```python
from build123d import *

# Parameters (mm, degrees)
BOSS_EXTRUDE1_DEPTH = 52.34
SKETCH2_R           = 2.2
CUT_EXTRUDE1_DEPTH  = 80
SKETCH3_R           = 49.6
CUT_EXTRUDE2_DEPTH  = 30


with BuildPart() as part:
    # Sketch1 → Boss-Extrude1 (new body)
    with BuildSketch(Plane(origin=(0, 0, 0), x_dir=(1, 0, 0), z_dir=(0, 1, 0))):
        with BuildLine():
            ThreePointArc((-53.971636069, -1.75), (-38.183766184, -38.183766184), (-1.75, -53.971636069))
            Line((-1.75, -53.971636069), (-1.75, -52.271636069))
            Line((-1.75, -52.271636069), (1.75, -52.271636069))
            Line((1.75, -52.271636069), (1.75, -53.971636069))
            ThreePointArc((1.75, -53.971636069), (38.183766184, -38.183766184), (53.971636069, -1.75))
            Line((53.971636069, -1.75), (52.271636069, -1.75))
            Line((52.271636069, -1.75), (52.271636069, 1.75))
            Line((52.271636069, 1.75), (53.971636069, 1.75))
            ThreePointArc((53.971636069, 1.75), (38.183766184, 38.183766184), (1.75, 53.971636069))
            Line((1.75, 53.971636069), (1.75, 52.271636069))
            Line((1.75, 52.271636069), (-1.75, 52.271636069))
            Line((-1.75, 52.271636069), (-1.75, 53.971636069))
            ThreePointArc((-1.75, 53.971636069), (-38.183766184, 38.183766184), (-53.971636069, 1.75))
            Line((-53.971636069, 1.75), (-52.271636069, 1.75))
            Line((-52.271636069, 1.75), (-52.271636069, -1.75))
            Line((-52.271636069, -1.75), (-53.971636069, -1.75))
        make_face()
    extrude(amount=BOSS_EXTRUDE1_DEPTH)

    # Sketch2 → Cut-Extrude1 (cut)
    with BuildSketch(Plane.XZ):
        with Locations(Location((0, 15.5, 0), (0, 0, 270))):
            Circle(SKETCH2_R)
        with Locations(Location((13.423393759, 7.75, 0), (0, 0, 270))):
            Circle(SKETCH2_R)
        with Locations(Location((13.423393759, -7.75, 0), (0, 0, 270))):
            Circle(SKETCH2_R)
        with Locations(Location((0, -15.5, 0), (0, 0, 270))):
            Circle(SKETCH2_R)
        with Locations(Location((-13.423393759, -7.75, 0), (0, 0, 270))):
            Circle(SKETCH2_R)
        with Locations(Location((-13.423393759, 7.75, 0), (0, 0, 270))):
            Circle(SKETCH2_R)
    extrude(amount=-CUT_EXTRUDE1_DEPTH, mode=Mode.SUBTRACT)

    # Sketch3 → Cut-Extrude2 (cut)
    with BuildSketch(Plane.XZ):
        with Locations(Location((0, 0, 0), (0, 0, 270))):
            Circle(SKETCH3_R)
    extrude(amount=-CUT_EXTRUDE2_DEPTH, mode=Mode.SUBTRACT)


solid = part.part
```
CAD build for the part. Positions are in the model's coordinates, mm. A direction names the side the tool comes from. Coordinates: 2 decimals unless noted, no trailing zeros. Order: outer loops, then holes, each group sorted by start corner. A loop starts at its lowest first (then second) coordinate and runs counter-clockwise, first axis right, second up.
(1) Saw through at A-A, the plane z = -7.75. Write the cut outline in (x, y), and give its area (3 significant figures).
Solution:
outline: (-53.44, 0) - (-48.99, 0) - (-48.99, 30) - (-15.62, 30) - (-15.62, 52.34) - (-53.44, 52.34) - close; (-11.22, 30) - (11.22, 30) - (11.22, 52.34) - (-11.22, 52.34) - close; (15.62, 30) - (48.99, 30) - (48.99, 0) - (53.44, 0) - (53.44, 52.34) - (15.62, 52.34) - close
area: 2,460 mm2
(2) Saw through at D-D, the plane z = 23. Write the cut outline in (x, y).
Solution:
outline: (-48.86, 0) - (-43.94, 0) - (-43.94, 30) - (43.94, 30) - (43.94, 0) - (48.86, 0) - (48.86, 52.34) - (-48.86, 52.34) - close
(3) Pin check, flat tips, straight feed: pin 1 Ø1.8 at (x, y) = (-0.5, 14.5) entering from +Z; pin 2 Ø4 at (y, z) = (42, 16.5) entering from -X; pin 3 Ø12 at (x, y) = (-18.5, 40.5) entering from +Z. Stop position of each tip, or through.
Solution:
pin 1: stops at z = 52.27
pin 2: stops at x = -52.02
pin 3: stops at z = 52.53
(4) Drill centre lines: L1, parallel to X at y = 14, z = 0; L2, parallel to X at y = 44, z = -7; L3, parallel to Z at x = 11.5, y = 45.5. Where is each one in solid material? Low to high.
Solution:
L1: x = -52.27 to -49.6, 49.6 to 52.27
L2: x = -53.54 to -15.49, -11.36 to 11.36, 15.49 to 53.54
L3: z = -52.76 to -8.82, -6.68 to 6.68, 8.82 to 52.76
(5) Which spindle directions (+Z, -Z, +X, -X, +Y, -Y) get a long thin tool onto all of the face, cutting with end or side? Do faces 1 (the face through (52.272, 26, 0)), 2 (the face through (0, 26, -52.272)), 3 (the face through (0, 26, 52.272)), 4 (the face through (14.9, 14.79, -47.31)). Say none if no direction does.
Solution:
face 1: +X, +Y, -Y
face 2: -Z, +Y, -Y
face 3: +Z, +Y, -Y
face 4: -Y
(6) Mould opens along X. For faces 5 (the face through (-11.568, 41.014, -8.933)), 6 (the face through (-48.23, 0, -12.25)), 7 (the face through (-52.272, 26, 0)), 8 (the face through (12.58, 41.01, -9.78)) say: released by +X, released by -X, zero draft, split by the parting line, or undercut.
Solution:
face 5: undercut
face 6: zero draft
face 7: released by -X
face 8: undercut
(7) Saw through at C-C, the plane y = 22. Write the cut outline in (x, z), and give its area (3 significant figures).
Solution:
outline: (-53.97, -1.75) arc R54 ccw to (-1.75, -53.97) - (-1.75, -52.27) - (1.75, -52.27) - (1.75, -53.97) arc R54 ccw to (53.97, -1.75) - (52.27, -1.75) - (52.27, 1.75) - (53.97, 1.75) arc R54 ccw to (1.75, 53.97) - (1.75, 52.27) - (-1.75, 52.27) - (-1.75, 53.97) arc R54 ccw to (-53.97, 1.75) - (-52.27, 1.75) - (-52.27, -1.75) - close; hole circle Ø99.2 at (0, 0)
area: 1,410 mm2
(8) Saw through at B-B, the plane y = 41.5. Write the cut outline in (x, z), and give its area (3 significant figures).
Solution:
outline: (-53.97, -1.75) arc R54 ccw to (-1.75, -53.97) - (-1.75, -52.27) - (1.75, -52.27) - (1.75, -53.97) arc R54 ccw to (53.97, -1.75) - (52.27, -1.75) - (52.27, 1.75) - (53.97, 1.75) arc R54 ccw to (1.75, 53.97) - (1.75, 52.27) - (-1.75, 52.27) - (-1.75, 53.97) arc R54 ccw to (-53.97, 1.75) - (-52.27, 1.75) - (-52.27, -1.75) - close; hole circle Ø4.4 at (-13.42, -7.75); hole circle Ø4.4 at (-13.42, 7.75); hole circle Ø4.4 at (0, -15.5); hole circle Ø4.4 at (0, 15.5); hole circle Ø4.4 at (13.42, -7.75); hole circle Ø4.4 at (13.42, 7.75)
area: 9,050 mm2
